Geometry: final body of the model. Coordinates: model frame, mm. Face numbers are marked on the shaded views. A direction names the side the tool comes from. Give positions to 0.01 mm unless a question says otherwise; leave off trailing zeros. Write each loop counter-clockwise with the first axis right and the second up, starting at its lowest first coordinate (ties: lowest second). Pieces come first, ordered by that corner, then holes.
```python
from build123d import *

# Parameters (mm, degrees)
SKETCH1_W           = 80
SKETCH1_H           = 38
BOSS_EXTRUDE1_DEPTH = 12
FILLET1_R           = 1
SKETCH3_W           = 57
SKETCH3_H           = 38
CUT_EXTRUDE1_DEPTH  = 4
SHELL1_T            = -3
CUT_EXTRUDE2_DEPTH  = 57
SKETCH5_R           = 0.9
SKETCH5_R_2         = 1.5
BOSS_EXTRUDE2_DEPTH = 1
SKETCH6_W           = 23
SKETCH6_H           = 38
CUT_EXTRUDE3_DEPTH  = 4
SKETCH7_W           = 9.5
SKETCH7_H           = 14
BOSS_EXTRUDE3_DEPTH = 8
SKETCH9_W           = 21
SKETCH9_H           = 34
CUT_EXTRUDE6_DEPTH  = 1
SKETCH8_W           = 3
SKETCH8_H           = 6.7
BOSS_EXTRUDE4_DEPTH = 9
CUT_EXTRUDE7_REACH  = 49.434
SKETCH10_R          = 1
SKETCH11_R          = 2
CUT_EXTRUDE8_DEPTH  = 2


with BuildPart() as part:
    # Sketch1 → Boss-Extrude1 (new, symmetric)
    with BuildSketch(Plane(origin=(0, 0, 0), x_dir=(1, 0, 0), z_dir=(0, 1, 0))):
        Rectangle(SKETCH1_W, SKETCH1_H)
    extrude(amount=BOSS_EXTRUDE1_DEPTH, both=True)

    # Fillet1
    fillet1_edges = [part.edges().sort_by_distance(p)[0] for p in [
        (-40, 12, 0),
        (0, 12, 19),
        (40, 12, 0),
        (0, -12, 19),
        (-40, -12, 0),
        (0, -12, -19),
        (40, -12, 0),
        (0, 12, -19),
        (40, 0, 19),
        (-40, 0, 19),
        (-40, 0, -19),
        (40, 0, -19),
    ]]
    fillet(fillet1_edges, radius=FILLET1_R)

    # Sketch3 → Cut-Extrude1 (cut)
    with BuildSketch(Plane(origin=(0, 12, 0), x_dir=(1, 0, 0), z_dir=(0, 1, 0))):
        with Locations((-11.5, 0)):
            Rectangle(SKETCH3_W, SKETCH3_H)
    extrude(amount=-CUT_EXTRUDE1_DEPTH, mode=Mode.SUBTRACT)

    # Shell1
    shell1_openings = [part.faces().sort_by_distance(p)[0] for p in [
        (17, 9.994969103, 0),
        (-11.494395734, 8, 0),
    ]]
    offset(amount=SHELL1_T, openings=shell1_openings, kind=Kind.INTERSECTION)

    # Sketch4 → Cut-Extrude2 (cut)
    with BuildSketch(Plane.ZY.offset(40)):
        Polygon((-18, 8), (-19, 8), (-19, 4), (-18, 4), (-17, 4), (-17, 6), (-18, 6), align=None)
    cut_extrude2 = extrude(amount=-CUT_EXTRUDE2_DEPTH, mode=Mode.SUBTRACT)

    # Mirror1: Cut-Extrude2 across plane
    add(cut_extrude2.mirror(Plane.XY), mode=Mode.SUBTRACT)

    # Sketch5 → Boss-Extrude2 (add)
    with BuildSketch(Plane(origin=(0, -9, 0), x_dir=(1, 0, 0), z_dir=(0, 1, 0))):
        with Locations(Location((-24, 0, 0), (0, 0, 270))):
            Circle(SKETCH5_R)
        with Locations(Location((-7.3, 0, 0), (0, 0, 270))):
            Circle(SKETCH5_R_2)
    extrude(amount=BOSS_EXTRUDE2_DEPTH)

    # Sketch6 → Cut-Extrude3 (cut)
    with BuildSketch(Plane(origin=(0, 12, 0), x_dir=(1, 0, 0), z_dir=(0, 1, 0))):
        with Locations((28.5, 0)):
            Rectangle(SKETCH6_W, SKETCH6_H)
    extrude(amount=-CUT_EXTRUDE3_DEPTH, mode=Mode.SUBTRACT)

    # Sketch7 → Boss-Extrude3 (add)
    with BuildSketch(Plane(origin=(0, -9, 0), x_dir=(1, 0, 0), z_dir=(0, 1, 0))):
        with Locations((26.75, 0)):
            Rectangle(SKETCH7_W, SKETCH7_H)
    extrude(amount=BOSS_EXTRUDE3_DEPTH)

    # Sketch9 → Cut-Extrude6 (cut)
    with BuildSketch(Plane(origin=(0, 8, 0), x_dir=(1, 0, 0), z_dir=(0, 1, 0))):
        with Locations((27.5, 0)):
            Rectangle(SKETCH9_W, SKETCH9_H)
    extrude(amount=-CUT_EXTRUDE6_DEPTH, mode=Mode.SUBTRACT)

    # Sketch8 → Boss-Extrude4 (add)
    with BuildSketch(Plane(origin=(0, -1, 0), x_dir=(1, 0, 0), z_dir=(0, 1, 0))):
        with Locations((28.5, 0)):
            Rectangle(SKETCH8_W, SKETCH8_H)
    extrude(amount=BOSS_EXTRUDE4_DEPTH)

    # Sketch10 → Cut-Extrude7 (cut, up to next)
    with BuildSketch(Plane(origin=(0, -9, 0), x_dir=(1, 0, 0), z_dir=(0, 1, 0)), mode=Mode.PRIVATE) as cut_extrude7_sk1:
        with Locations(Location((28.5, 11, 0), (0, 0, 270))):
            Circle(SKETCH10_R)
    cut_extrude7_tool1 = extrude(cut_extrude7_sk1.sketch, amount=-CUT_EXTRUDE7_REACH, mode=Mode.PRIVATE) & part.part
    # Sketch10 → Cut-Extrude7 (cut, up to next)
    with BuildSketch(Plane(origin=(0, -9, 0), x_dir=(1, 0, 0), z_dir=(0, 1, 0)), mode=Mode.PRIVATE) as cut_extrude7_sk2:
        with Locations(Location((28.5, -11, 0), (0, 0, 270))):
            Circle(SKETCH10_R)
    cut_extrude7_tool2 = extrude(cut_extrude7_sk2.sketch, amount=-CUT_EXTRUDE7_REACH, mode=Mode.PRIVATE) & part.part
    add(cut_extrude7_tool1.solids().sort_by_distance((28.5, -9, -11))[0], mode=Mode.SUBTRACT)
    add(cut_extrude7_tool2.solids().sort_by_distance((28.5, -9, 11))[0], mode=Mode.SUBTRACT)

    # Sketch11 → Cut-Extrude8 (cut)
    with BuildSketch(Plane.XZ.offset(12)):
        with Locations(Location((28.5, -11, 0), (0, 0, 270))):
            Circle(SKETCH11_R)
        with Locations(Location((28.5, 11, 0), (0, 0, 270))):
            Circle(SKETCH11_R)
    extrude(amount=-CUT_EXTRUDE8_DEPTH, mode=Mode.SUBTRACT)


solid = part.part
```
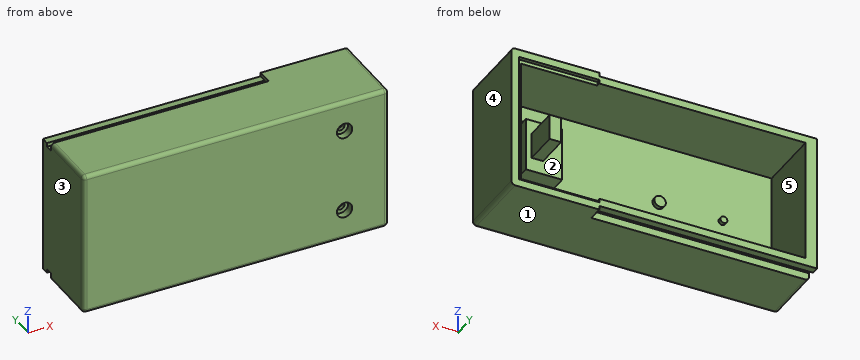
Item 1: Section A-A, the plane y = -5. Return the cut outline in (x, z), plus the area to 3 significant figures.
Found:
outline: (-40, -18) arc R1 ccw to (-39, -19) - (39, -19) arc R1 ccw to (40, -18) - (40, 18) arc R1 ccw to (39, 19) - (-39, 19) arc R1 ccw to (-40, 18) - close; (22, -7) - (31.5, -7) - (31.5, 7) - (22, 7) - close; hole (-37, -16) - (37, -16) - (37, 16) - (-37, 16) - close
area: 804 mm2
Item 2: Section D-D, the plane x = -7.3. Return the cut outline in (y, z), plus the area to 3 significant figures.
Found:
outline: (-12, -18) arc R1 ccw to (-11, -19) - (4, -19) - (4, -17) - (6, -17) - (6, -18) - (8, -18) - (8, -16) - (-9, -16) - (-9, -1.5) - (-8, -1.5) - (-8, 1.5) - (-9, 1.5) - (-9, 16) - (8, 16) - (8, 18) - (6, 18) - (6, 17) - (4, 17) - (4, 19) - (-11, 19) arc R1 ccw to (-12, 18) - close
area: 207 mm2
Item 3: Section C-C, the plane z = -4.5. Return the cut outline in (x, y), plus the area to 3 significant figures.
Found:
outline: (-40, -11) arc R1 ccw to (-39, -12) - (39, -12) arc R1 ccw to (40, -11) - (40, 8) - (38, 8) - (38, 7) - (37, 7) - (37, -9) - (31.5, -9) - (31.5, -1) - (22, -1) - (22, -9) - (-37, -9) - (-37, 8) - (-40, 8) - close
area: 417 mm2
Item 4: Pin query (flat end, axial travel): pin 1 Ø5 at (x, z) = (-7.5, -6.5) entering from +Y; pin 2 Ø1.6 at (x, y) = (-21.5, 7.5) entering from -Z. Return the tip coordinate at first contact, or that it passes through.
Found:
pin 1: stops at y = -9
pin 2: stops at z = -18
Item 5: Reachability of the marked faces 4 and 5 from +Z, -Z, +X, -X, +Y, -Y: full face, straight path, thin tool, end or side. Return the list, or none.
Found:
face 4: +Z, -Z, +X, +Y, -Y
face 5: +Y
Item 6: Line query: L1, parallel to X at y = -1.25, z = -5.5; L2, parallel to Z at x = -3, y = 0; L3, parallel to X at y = -10.55, z = -11. Output: solid intervals per line, ascending.
Found:
L1: x = -40 to -37, 22 to 31.5, 37 to 40
L2: z = -19 to -16, 16 to 19
L3: x = -40 to 26.5, 30.5 to 40
Item 7: Pull-direction query (Z, two-part tool) for the marked faces 1, 2 and 3; classes: +Z half, -Z half, draft (parallel to the pull), parting line (faces both ways), or undercut.
Found:
face 1: -Z half
face 2: undercut
face 3: draft
Item 8: Section B-B, the plane z = -11. Return the cut outline in (x, y).
Found:
outline: (-40, -11) arc R1 ccw to (-39, -12) - (26.5, -12) - (26.5, -10) - (27.5, -10) - (27.5, -9) - (-37, -9) - (-37, 8) - (-40, 8) - close; (29.5, -10) - (30.5, -10) - (30.5, -12) - (39, -12) arc R1 ccw to (40, -11) - (40, 8) - (38, 8) - (38, 7) - (37, 7) - (37, -9) - (29.5, -9) - close
